```python
from build123d import *

# Parameters (mm, degrees)
SKETCH1_W           = 38.1
SKETCH1_H           = 57.15
BOSS_EXTRUDE1_DEPTH = 10.16
SHELL1_T            = -2.54
SKETCH3_R           = 1.651
SKETCH3_R_2         = 3.175
CUT_EXTRUDE1_DEPTH  = 27.94


with BuildPart() as part:
    # Sketch1 → Boss-Extrude1 (new body)
    with BuildSketch(Plane(origin=(0, 0, 0), x_dir=(1, 0, 0), z_dir=(0, 1, 0))):
        with Locations((19.05, 28.575)):
            Rectangle(SKETCH1_W, SKETCH1_H)
    extrude(amount=BOSS_EXTRUDE1_DEPTH)

    # Shell1
    shell1_openings = [part.faces().sort_by_distance(p)[0] for p in [
        (19.05, 10.16, -28.575),
    ]]
    offset(amount=SHELL1_T, openings=shell1_openings, kind=Kind.INTERSECTION)

    # Sketch3 → Cut-Extrude1 (cut)
    with BuildSketch(Plane.XZ):
        with Locations(Location((19.05, -38.1, 0), (0, 0, 270))):
            Circle(SKETCH3_R)
        with Locations(Location((19.05, -20.32, 0), (0, 0, 270))):
            Circle(SKETCH3_R_2)
    extrude(amount=-CUT_EXTRUDE1_DEPTH, mode=Mode.SUBTRACT)


solid = part.part
```
Geometry: final body of the model. Coordinates: model frame, mm. A direction names the side the tool comes from. Round coordinates to 2 decimals unless told otherwise and drop trailing zeros. Loops run counter-clockwise (first coordinate to the right, second up) from the corner with the lowest first, then second, coordinate; pieces in that order, holes last. Notation, with made-up numbers: (81.5, -22.75) -> (113.5, -22.75) arc R16 cw to (113.5, -2.75) -> close; hole circle Ø2 at (-10, -13). An arc over 180 degrees is marked (long way). Use one line per item in the form item = value. Start each with the question number.
1) Access query for faces 5 (the cylindrical face through (15.95, 1.25, -19.63)), 6 (the flat face through (2.54, 6, -28)). Directions: +Z, -Z, +X, -X, +Y, -Y. A direction counts if a zero-diameter tool reaches every point of the face in a straight line with its end or side. Return the directions, or none.
2) Section A-A on x = 19.05. Output: boundary loops of the cut face in (y, z) (3 decimals).
3) Line query: L1, parallel to X at y = 1.75, z = -20.32 (3 decimals); L2, parallel to Z at x = 12, y = 5; L3, parallel to X at y = 4.5, z = -46.5. Output: solid intervals per line, ascending.
4) Section C-C on y = 5.75. Output: boundary loops of the cut face in (x, z).
5) First-contact query: P1, Ø10, axis at x = 26.5, z = -32, coming from the +Y side. Flat tip, straight axial feed; report the tip coordinate or a pass-through.
6) Draft query along Z for faces 1 (the flat face through (19, 2.54, -29)), 2 (the flat face through (19, 5, 0)), 3 (the flat face through (38.1, 5, -28)), 4 (the flat face through (19, 5, -57.15)). Return one class per face: released by +Z, released by -Z, zero draft, split by the parting line, or undercut.
7) Section D-D on z = -45.5. Output: boundary loops of the cut face in (x, y).
8) Section B-B on z = -38.1. Output: boundary loops of the cut face in (x, y), then the cut area to 3 significant figures.
Response:
q1.face_5 = +Y, -Y
q1.face_6 = +Y
q2.outline = (0, -57.15) -> (10.16, -57.15) -> (10.16, -54.61) -> (2.54, -54.61) -> (2.54, -39.751) -> (0, -39.751) -> close; (0, -36.449) -> (2.54, -36.449) -> (2.54, -23.495) -> (0, -23.495) -> close; (0, -17.145) -> (2.54, -17.145) -> (2.54, -2.54) -> (10.16, -2.54) -> (10.16, 0) -> (0, 0) -> close
q3.L1 = 0 to 15.875, 22.225 to 38.1
q3.L2 = -57.15 to -54.61, -2.54 to 0
q3.L3 = 0 to 2.54, 35.56 to 38.1
q4.outline = (0, -57.15) -> (38.1, -57.15) -> (38.1, 0) -> (0, 0) -> close; hole (2.54, -54.61) -> (35.56, -54.61) -> (35.56, -2.54) -> (2.54, -2.54) -> close
q5.P1 = 2.54
q6.face_1 = undercut
q6.face_2 = released by +Z
q6.face_3 = zero draft
q6.face_4 = released by -Z
q7.outline = (0, 0) -> (38.1, 0) -> (38.1, 10.16) -> (35.56, 10.16) -> (35.56, 2.54) -> (2.54, 2.54) -> (2.54, 10.16) -> (0, 10.16) -> close
q8.outline = (0, 0) -> (17.4, 0) -> (17.4, 2.54) -> (2.54, 2.54) -> (2.54, 10.16) -> (0, 10.16) -> close; (20.7, 0) -> (38.1, 0) -> (38.1, 10.16) -> (35.56, 10.16) -> (35.56, 2.54) -> (20.7, 2.54) -> close
q8.area = 127 mm^2
